The figure shows three views and two pictorial views of one solid part (mm, origin at its lowest corner). Answer the questions. A direction names the side the tool comes from. Coordinates: 2 decimals unless noted, no trailing zeros. Write each loop counter-clockwise with the first axis right and the second up, starting at its lowest first coordinate (ties: lowest second). Pieces come first, ordered by that corner, then holes. Notation, with made-up numbers: (65.5, 88) - (86.5, 88) arc R24 ccw to (86.5, 125) - close; hole circle Ø3 at (49, -40). An arc over 180 degrees is marked (long way). Use a Markdown table: item, result. Add a question column.
(1) Given pin 1 Ø4.5 at (y, z) = (4, 2) entering from -X; pin 2 Ø1.6 at (x, z) = (3.5, 12) entering from -Y; pin 3 Ø1.9 at (x, y) = (4.5, 5) entering from -Z; pin 4 Ø4.5 at (x, z) = (2.5, 15) entering from +Y, each flat-ended and moving along its own axis, determine where each tip first touches the part or whether it passes through.
(2) For a pull along X with two mould halves and no side action, classify the marked faces 5, 6, 7 and 8 as released by +X, released by -X, zero draft, split by the parting line, or undercut.
(3) A tool of negligible diameter and unlimited length cuts with its end or side. For the marked faces 1, 2, 3 and 4, from which of +Z, -Z, +X, -X, +Y, -Y can it reach the whole face along a straight path? Write none if from no direction.
(4) Find the intervals of material crossed by line 1 (X direction, y = 6, z = 2); line 2 (X direction, y = 1.25, z = 15.75), in increasing order. Write a range as from..to.
(5) The part is cut by section A-A, the plane x = 5.25. Give the vertices of the cut face in (y, z).
(6) The part is cut by section C-C, the plane z = 1.5. Give the vertices of the cut face in (x, y).
(7) The part is cut by section D-D, the plane z = 11.75. Give the vertices of the cut face in (x, y), then the cut area to 3 significant figures.
(8) The part is cut by section B-B, the plane y = 6. Give the vertices of the cut face in (x, z), then the cut area to 3 significant figures.
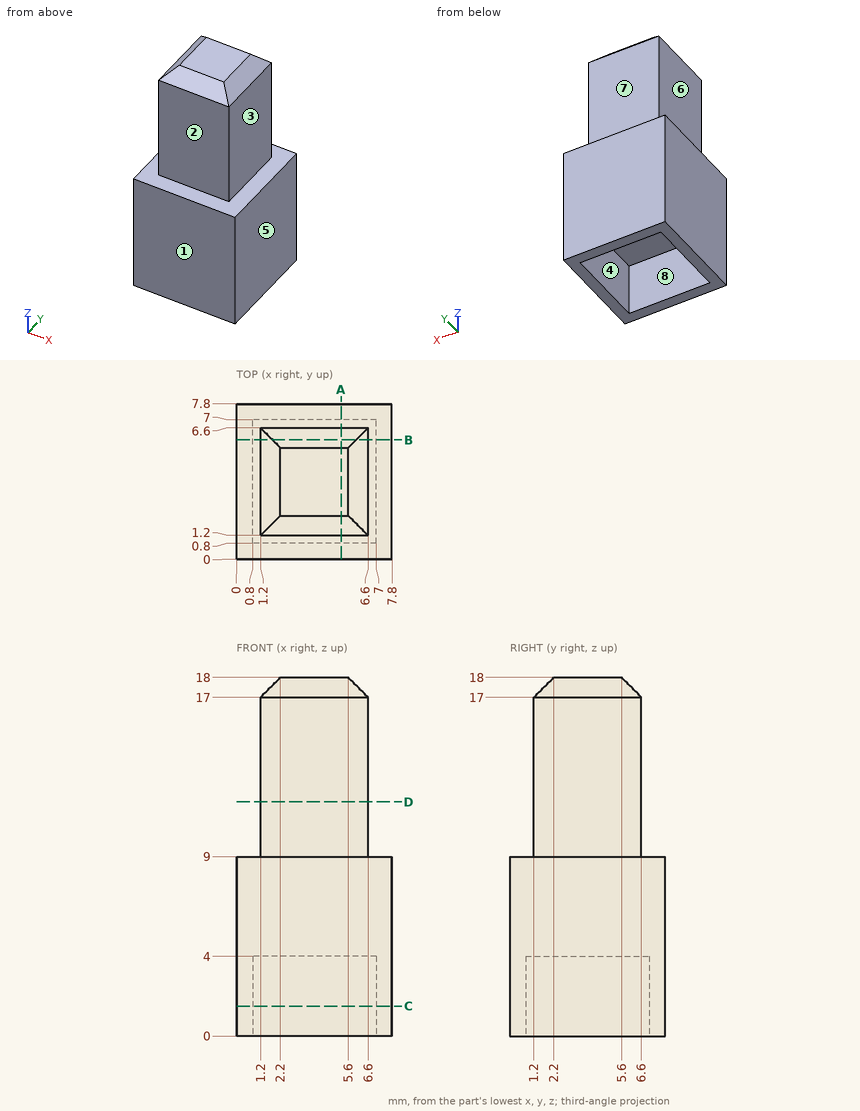
Model answer:
| question | item | result |
|---|---|---|
| 1 | pin 1 | x = 0 |
| 1 | pin 2 | y = 1.2 |
| 1 | pin 3 | z = 4 |
| 1 | pin 4 | y = 6.6 |
| 2 | face 5 | released by +X |
| 2 | face 6 | released by -X |
| 2 | face 7 | zero draft |
| 2 | face 8 | undercut |
| 3 | face 1 | +Z, -Z, +X, -X, -Y |
| 3 | face 2 | +Z, +X, -X, -Y |
| 3 | face 3 | +Z, +X, +Y, -Y |
| 3 | face 4 | -Z |
| 4 | line 1 | 0..0.8, 7..7.8 |
| 4 | line 2 | 1.2..6.6 |
| 5 | outline | (0, 0) - (0.8, 0) - (0.8, 4) - (7, 4) - (7, 0) - (7.8, 0) - (7.8, 9) - (6.6, 9) - (6.6, 17) - (5.6, 18) - (2.2, 18) - (1.2, 17) - (1.2, 9) - (0, 9) - close |
| 6 | outline | (0, 0) - (7.8, 0) - (7.8, 7.8) - (0, 7.8) - close; hole (0.8, 0.8) - (7, 0.8) - (7, 7) - (0.8, 7) - close |
| 7 | outline | (1.2, 1.2) - (6.6, 1.2) - (6.6, 6.6) - (1.2, 6.6) - close |
| 7 | area | 29.2 mm^2 |
| 8 | outline | (0, 0) - (0.8, 0) - (0.8, 4) - (7, 4) - (7, 0) - (7.8, 0) - (7.8, 9) - (6.6, 9) - (6.6, 17) - (6, 17.6) - (1.8, 17.6) - (1.2, 17) - (1.2, 9) - (0, 9) - close |
| 8 | area | 91.5 mm^2 |
